Verification items for the finished model (mm, model axes). Face numbers are marked on the shaded views. A direction names the side the tool comes from. Round coordinates to 2 decimals unless told otherwise and drop trailing zeros. Write each loop counter-clockwise with the first axis right and the second up, starting at its lowest first coordinate (ties: lowest second). Pieces come first, ordered by that corner, then holes. Notation, with made-up numbers: M -35,20 L 21,20 A30 cw 21,47 Z; hole C 43,-14.75 d2. An arc over 180 degrees is marked long. Answer in a Markdown table with one row per item. Add a question column.
1. Go/stop test with flat-tipped pins: pin 1 Ø1 at (x, z) = (2.5, 3) entering from +Y; pin 2 Ø4 at (y, z) = (17.5, -1.5) entering from -X; pin 3 Ø1.5 at (y, z) = (72.5, 0.5) entering from +X. Record where each tip stops, or that it passes through.
2. Set-up check for the marked faces 1 and 2: record each of +Z, -Z, +X, -X, +Y, -Y from which the full face is reachable in a straight line by a thin tool's end or side.
3. Sectioned sample at C-C on y = 17.5. Record the cut outline in (x, z) (3 decimals), plus the area to 3 significant figures.
4. Material ranges on probe 1 along Y at (x, z) = (-2.25, 1.5); probe 2 along X at (y, z) = (32.5, 0.25); probe 3 along Z at (x, y) = (1.5, 62), recorded low to high.
5. Sectioned sample at B-B on y = 77. Record the cut outline in (x, z) (3 decimals), plus the area to 3 significant figures.
6. Sectioned sample at A-A on x = 0. Record the cut outline in (y, z), plus the area to 3 significant figures.
```python
from build123d import *

# Parameters (mm, degrees)
BOSS_EXTRUDE1_DEPTH = 7
SKETCH2_R           = 2.95
BOSS_EXTRUDE2_DEPTH = 160
SKETCH5_R           = 2.95
SKETCH4_R           = 3.95
BOSS_EXTRUDE3_DEPTH = 7


with BuildPart() as part:
    # Sketch1 → Boss-Extrude1 (new body)
    with BuildSketch(Plane(origin=(0, 0, 0), x_dir=(1, 0, 0), z_dir=(0, 1, 0))):
        Polygon((1.475, -2.554774941), (2.95, 0), (1.475, 2.554774941), (-1.475, 2.554774941), (-2.95, 0), (-1.475, -2.554774941), align=None)
    extrude(amount=BOSS_EXTRUDE1_DEPTH)

    # Sketch2 → Boss-Extrude2 (add)
    with BuildSketch(Plane(origin=(0, 7, 0), x_dir=(1, 0, 0), z_dir=(0, 1, 0))):
        with Locations(Location((0, 0, 0), (0, 0, 60))):
            Circle(SKETCH2_R)
    extrude(amount=BOSS_EXTRUDE2_DEPTH)

    # Sketch5 → Loft1 section 0
    with BuildSketch(Plane.XZ.offset(-7)):
        Circle(SKETCH5_R)
    # Sketch4 → Loft1 section 1
    with BuildSketch(Plane(origin=(0, 27, 0), x_dir=(-1, 0, 0), z_dir=(0, -1, 0))):
        Circle(SKETCH4_R)
    loft()

    # Sketch6 → Boss-Extrude3 (add)
    with BuildSketch(Plane(origin=(0, 167, 0), x_dir=(1, 0, 0), z_dir=(0, 1, 0))):
        Polygon((1.475, -2.554774941), (2.95, 0), (1.475, 2.554774941), (-1.475, 2.554774941), (-2.95, 0), (-1.475, -2.554774941), align=None)
    extrude(amount=BOSS_EXTRUDE3_DEPTH)


solid = part.part
```
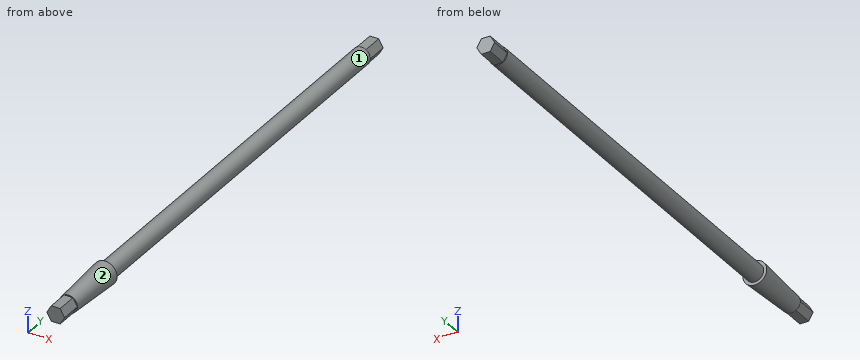
Geometry check:
| question | item | result |
|---|---|---|
| 1 | pin 1 | stops at y = 27 |
| 1 | pin 2 | stops at x = -3.55 |
| 1 | pin 3 | stops at x = 2.95 |
| 2 | face 1 | +Y |
| 2 | face 2 | -Y |
| 3 | outline | C 0,0 d6.95 |
| 3 | area | 37.9 mm2 |
| 4 | probe 1 | y = 7 to 167 |
| 4 | probe 2 | x = -2.94 to 2.94 |
| 4 | probe 3 | z = -2.54 to 2.54 |
| 5 | outline | C 0,0 d5.9 |
| 5 | area | 27.3 mm2 |
| 6 | outline | M 0,-2.55 L 7,-2.55 L 7,-2.95 L 27,-3.95 L 27,-2.95 L 167,-2.95 L 167,-2.55 L 174,-2.55 L 174,2.55 L 167,2.55 L 167,2.95 L 27,2.95 L 27,3.95 L 7,2.95 L 7,2.55 L 0,2.55 Z |
| 6 | area | 1,040 mm2 |
